The model under review builds one solid part; all positions refer to its coordinate system, in mm. A direction names the side the tool comes from. Coordinates: 2 decimals unless noted, no trailing zeros. Loops run counter-clockwise (first coordinate to the right, second up) from the corner with the lowest first, then second, coordinate; pieces in that order, holes last. Notation, with made-up numbers: M 63,5 L 87,5 A21 ccw 87,29 Z; hole C 71,-17.75 d7. An arc over 180 degrees is marked long. Write item = value, one per line. Start each with the question number.
Q1. We need section A-A on z = -9. Give the boundary of the cut face in (x, y) (3 decimals).
Q2. We need section B-B on x = -21. Give the boundary of the cut face in (y, z).
Q3. We need section D-D on z = -3.25. Give the boundary of the cut face in (x, y).
Q4. Clearance check with a flat-ended pin moving along its axis: pin 1 Ø12 at (x, z) = (-17, 0) entering from +Y. State where the tip first meets the part, or that it passes through.
Q5. We need section C-C on y = 3. Give the boundary of the cut face in (x, z).
Q6. For faces 1 (the face through (-10, 5, 0)), 2 (the face through (0, 0, 0)), 3 (the face through (-19, 2, 0)), list the 3-axis set-ups (+Z, -Z, +X, -X, +Y, -Y) from which the entire face can be reached by the end or side of a thin tool; tool diameter is ignored.
Q7. Wall thickness on probe 1 along X at (y, z) = (2, 9); probe 2 along X at (y, z) = (4.25, -9); probe 3 along Z at (x, y) = (-1, 4.25): over which ranges is each line inside the solid? List them lowest first.
from build123d import *

# Parameters (mm, degrees)
SKETCH1_W                      = 50
SKETCH1_H                      = 30
BOSS_EXTRUDE1_DEPTH            = 7
SKETCH2_W                      = 15
SKETCH2_H                      = 30
CUT_EXTRUDE1_DEPTH             = 3.5
CUT_EXTRUDE2_DEPTH             = 4.5
M3_CLEARANCE_HOLE1_D           = 3.2
M3_CLEARANCE_HOLE1_CSINK_D     = 3.25
M3_CLEARANCE_HOLE1_CSINK_ANGLE = 90


with BuildPart() as part:
    # Sketch1 → Boss-Extrude1 (new body)
    with BuildSketch(Plane(origin=(0, 0, 0), x_dir=(1, 0, 0), z_dir=(0, 1, 0))):
        Rectangle(SKETCH1_W, SKETCH1_H)
    extrude(amount=BOSS_EXTRUDE1_DEPTH)

    # Sketch2 → Cut-Extrude1 (cut)
    with BuildSketch(Plane(origin=(0, 7, 0), x_dir=(1, 0, 0), z_dir=(0, 1, 0))):
        with Locations((-17.5, 0)):
            Rectangle(SKETCH2_W, SKETCH2_H)
    extrude(amount=-CUT_EXTRUDE1_DEPTH, mode=Mode.SUBTRACT)

    # Sketch3 → Cut-Extrude2 (cut, through all)
    with BuildSketch(Plane(origin=(0, 3.5, 0), x_dir=(1, 0, 0), z_dir=(0, 1, 0))):
        with BuildLine():
            Line((-19, 10), (-19, -10))
            ThreePointArc((-19, -10), (-21, -12), (-23, -10))
            Line((-23, -10), (-23, 10))
            ThreePointArc((-23, 10), (-21, 12), (-19, 10))
        make_face()
    extrude(amount=-CUT_EXTRUDE2_DEPTH, mode=Mode.SUBTRACT)

    # M3 Clearance Hole1 (through all)
    with Locations(Plane(origin=(0, 7, 0), x_dir=(1, 0, 0), z_dir=(0, 1, 0))):
        with Locations((-1, 9), (-1, -9), (19, 9), (19, -9)):
            CounterSinkHole(M3_CLEARANCE_HOLE1_D / 2, M3_CLEARANCE_HOLE1_CSINK_D / 2, counter_sink_angle=M3_CLEARANCE_HOLE1_CSINK_ANGLE)


solid = part.part
Returned:
q1.outline = M -25,0 L -23,0 L -23,3.5 L -25,3.5 Z; M -19,0 L -2.6,0 L -2.6,6.975 L -2.625,7 L -10,7 L -10,3.5 L -19,3.5 Z; M 0.6,0 L 17.4,0 L 17.4,6.975 L 17.375,7 L 0.625,7 L 0.6,6.975 Z; M 20.6,0 L 25,0 L 25,7 L 20.625,7 L 20.6,6.975 Z
q2.outline = M 0,-15 L 3.5,-15 L 3.5,-12 L 0,-12 Z; M 0,12 L 3.5,12 L 3.5,15 L 0,15 Z
q3.outline = M -25,0 L -23,0 L -23,3.5 L -25,3.5 Z; M -19,0 L 25,0 L 25,7 L -10,7 L -10,3.5 L -19,3.5 Z
q4.pin_1 = 3.5
q5.outline = M -25,-15 L 25,-15 L 25,15 L -25,15 Z; hole M -23,-10 A2 ccw -19,-10 L -19,10 A2 ccw -23,10 Z; hole C -1,-9 d3.2; hole C -1,9 d3.2; hole C 19,-9 d3.2; hole C 19,9 d3.2
q6.face_1 = +Z, -Z, -X, +Y
q6.face_2 = +Z, -Z, +X, -X, -Y
q6.face_3 = +Y, -Y
q7.probe_1 = -25 to -23, -19 to -2.6, 0.6 to 17.4, 20.6 to 25
q7.probe_2 = -10 to -2.6, 0.6 to 17.4, 20.6 to 25
q7.probe_3 = -15 to -10.6, -7.4 to 7.4, 10.6 to 15
